Drawing for the job (mm, zero at the part's lowest x, y, z). A direction names the side the tool comes from. Give positions to 0.01 mm unless a question says otherwise; leave off trailing zeros. Order: outer loops, then holes, each group sorted by start corner. A loop starts at its lowest first (then second) coordinate and runs counter-clockwise, first axis right, second up. Notation, with made-up numbers: (75, 76.25) -> (114, 76.25) arc R15 ccw to (114, 80.25) -> close; hole circle Ø9 at (23.25, 48.5). An arc over 180 degrees is marked (long way). One line per item, written item: value. Start each with the question number.
(1) Probe line 1 (Z direction, x = 552, y = 29); line 2 (X direction, y = 59, z = 178.5); line 3 (Z direction, x = 440, y = 60.5). List the from-to ranges inside material, lowest first.
(2) Saw through at D-D on y = 28.5. Give the cut face in (x, z).
(3) Saw through at C-C on z = 89. Give the cut face in (x, y).
(4) Two-plate mould, pull along X, no slides. Class the marked faces 3, 4 and 5: +X half, -X half, draft (parallel to the pull), parting line (faces both ways), or undercut.
(5) Pin check, flat tips, straight feed: pin 1 (4 mm diameter, centred on x = 112.5, z = 271.5, fed in from +Y); pin 2 (15 mm diameter, centred on x = 566.5, y = 30.5, fed in from -Z). Stop position of each tip, or through.
(6) Saw through at B-B on x = 209. Give the cut face in (y, z).
(7) Which spindle directions (+Z, -Z, +X, -X, +Y, -Y) get a long thin tool onto all of the face, cutting with end or side? Do the marked faces 1 and 2. Say none if no direction does.
(8) Saw through at A-A on y = 62. Give the cut face in (x, z), plus the area to 3 significant figures.
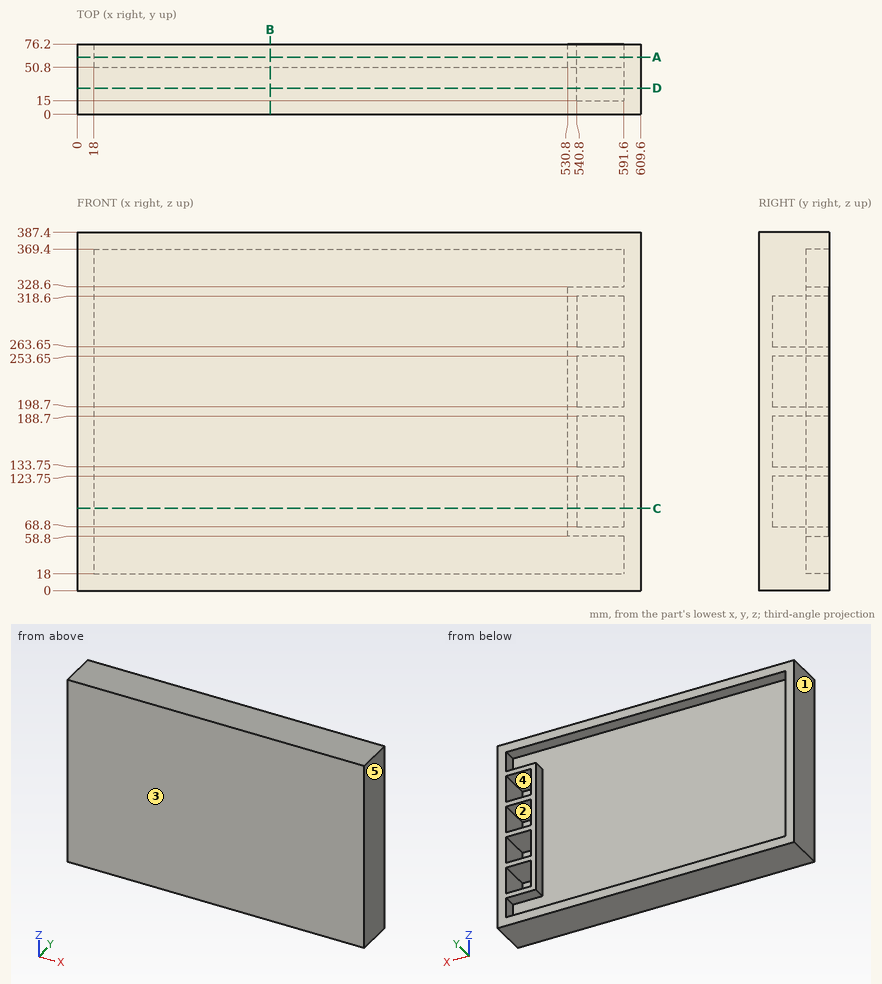
Results below:
1. line 1: z = 0 to 68.8, 123.75 to 133.75, 188.7 to 198.7, 253.65 to 263.65, 318.6 to 387.4
1. line 2: x = 0 to 18, 530.8 to 540.8, 591.6 to 609.6
1. line 3: z = 0 to 18, 369.4 to 387.4
2. outline: (0, 0) -> (609.6, 0) -> (609.6, 387.4) -> (0, 387.4) -> close; hole (540.8, 68.8) -> (591.6, 68.8) -> (591.6, 123.75) -> (540.8, 123.75) -> close; hole (540.8, 133.75) -> (591.6, 133.75) -> (591.6, 188.7) -> (540.8, 188.7) -> close; hole (540.8, 198.7) -> (591.6, 198.7) -> (591.6, 253.65) -> (540.8, 253.65) -> close; hole (540.8, 263.65) -> (591.6, 263.65) -> (591.6, 318.6) -> (540.8, 318.6) -> close
3. outline: (0, 0) -> (609.6, 0) -> (609.6, 76.2) -> (591.6, 76.2) -> (591.6, 15) -> (540.8, 15) -> (540.8, 76.2) -> (530.8, 76.2) -> (530.8, 50.8) -> (18, 50.8) -> (18, 76.2) -> (0, 76.2) -> close
4. face 3: draft
4. face 4: undercut
4. face 5: +X half
5. pin 1: stops at y = 50.8
5. pin 2: stops at z = 0
6. outline: (0, 0) -> (76.2, 0) -> (76.2, 18) -> (50.8, 18) -> (50.8, 369.4) -> (76.2, 369.4) -> (76.2, 387.4) -> (0, 387.4) -> close
7. face 1: +Z, -Z, -X, +Y, -Y
7. face 2: +Y
8. outline: (0, 0) -> (609.6, 0) -> (609.6, 387.4) -> (0, 387.4) -> close; hole (18, 18) -> (591.6, 18) -> (591.6, 58.8) -> (530.8, 58.8) -> (530.8, 328.6) -> (591.6, 328.6) -> (591.6, 369.4) -> (18, 369.4) -> close; hole (540.8, 68.8) -> (591.6, 68.8) -> (591.6, 123.75) -> (540.8, 123.75) -> close; hole (540.8, 133.75) -> (591.6, 133.75) -> (591.6, 188.7) -> (540.8, 188.7) -> close; hole (540.8, 198.7) -> (591.6, 198.7) -> (591.6, 253.65) -> (540.8, 253.65) -> close; hole (540.8, 263.65) -> (591.6, 263.65) -> (591.6, 318.6) -> (540.8, 318.6) -> close
8. area: 39,800 mm²
